from build123d import *

# Parameters (mm, degrees)
SKETCH1_R                = 49.5
BOSS_EXTRUDE1_DEPTH      = 3.18
CUT_EXTRUDE1_START       = -3.18
CUT_EXTRUDE1_DEPTH       = 3.18
CIRPATTERN1_COUNT        = 20
CUT_EXTRUDE2_DEPTH       = 70.51411196
FILLET2_R                = 1
CIRPATTERN2_COUNT        = 6
FILLET2_OF_CIRPATTERN2_R = 1
CUT_EXTRUDE3_DEPTH       = 70.51411196
SKETCH7_R                = 1
CUT_EXTRUDE4_DEPTH       = 70.51411196
CIRPATTERN3_COUNT        = 6


with BuildPart() as part:
    # Sketch1 → Boss-Extrude1 (new body)
    with BuildSketch(Plane.XY):
        with Locations(Location((0, 0, 0), (0, 0, 180))):
            Circle(SKETCH1_R)
    extrude(amount=BOSS_EXTRUDE1_DEPTH)

    # Sketch2 → Cut-Extrude1 (cut)
    with BuildSketch(Plane.XY.offset(3.18).offset(CUT_EXTRUDE1_START)):
        with BuildLine():
            ThreePointArc((-6.261015826, 49.102440681), (-3.38164679, 44.537884692), (-1.984798992, 39.324943712))
            ThreePointArc((-1.984798992, 39.324943712), (0, 39.375), (1.984798992, 39.324943712))
            ThreePointArc((1.984798992, 39.324943712), (3.38164679, 44.537884692), (6.261015826, 49.102440681))
            ThreePointArc((6.261015826, 49.102440681), (0, 49.5), (-6.261015826, 49.102440681))
        make_face()
    cut_extrude1 = extrude(amount=CUT_EXTRUDE1_DEPTH, mode=Mode.SUBTRACT)

    # CirPattern1: Cut-Extrude1 ×20 about axis
    cirpattern1_axis = Axis((0, 0, 0), (0, 0, 1))
    for i in range(1, CIRPATTERN1_COUNT):
        add(cut_extrude1.rotate(cirpattern1_axis, i * 360 / CIRPATTERN1_COUNT), mode=Mode.SUBTRACT)

    # Sketch3 → Cut-Extrude2 (cut, through all)
    with BuildSketch(Plane.XY.offset(3.18)):
        Polygon((6.06887616, 7.947876581), (29.56119168, 16.498380165), (14.619379743, 31.440192101), align=None)
    cut_extrude2 = extrude(amount=-CUT_EXTRUDE2_DEPTH, mode=Mode.SUBTRACT)

    # Fillet2
    fillet2_edges = [part.edges().sort_by_distance(p)[0] for p in [
        (29.56119168, 16.498380165, 1.59),
        (6.06887616, 7.947876581, 1.59),
        (14.619379743, 31.440192101, 1.59),
    ]]
    fillet(fillet2_edges, radius=FILLET2_R)

    # CirPattern2: Cut-Extrude2 ×6 about axis
    cirpattern2_axis = Axis((0, 0, 0), (0, 0, 1))
    for i in range(1, CIRPATTERN2_COUNT):
        add(cut_extrude2.rotate(cirpattern2_axis, i * 360 / CIRPATTERN2_COUNT), mode=Mode.SUBTRACT)

    # Fillet2 of CirPattern2
    fillet2_of_cirpattern2_edges = [part.edges().sort_by_distance(p)[0] for p in [
        (0.492579496, 33.849933043, 1.59),
        (-3.848624946, 9.229739218, 1.59),
        (-19.918315188, 28.380850296, 1.59),
        (-29.068612184, 17.351552878, 1.59),
        (-9.917501106, 1.281862636, 1.59),
        (-34.537694931, -3.059341805, 1.59),
        (-29.56119168, -16.498380165, 1.59),
        (-6.06887616, -7.947876581, 1.59),
        (-14.619379743, -31.440192101, 1.59),
        (-0.492579496, -33.849933043, 1.59),
        (3.848624946, -9.229739218, 1.59),
        (19.918315188, -28.380850296, 1.59),
        (29.068612184, -17.351552878, 1.59),
        (9.917501106, -1.281862636, 1.59),
        (34.537694931, 3.059341805, 1.59),
    ]]
    fillet(fillet2_of_cirpattern2_edges, radius=FILLET2_OF_CIRPATTERN2_R)

    # Sketch5 → Cut-Extrude3 (cut, through all)
    with BuildSketch(Plane.XY.offset(3.18)):
        with BuildLine():
            Line((-1.322875656, 1.5), (1.322875656, 1.5))
            ThreePointArc((1.322875656, 1.5), (0, -2), (-1.322875656, 1.5))
        make_face()
    extrude(amount=-CUT_EXTRUDE3_DEPTH, mode=Mode.SUBTRACT)

    # Sketch7 → Cut-Extrude4 (cut, through all)
    with BuildSketch(Plane(origin=(0, 0, 0), x_dir=(-1, 0, 0), z_dir=(0, 0, -1))):
        with Locations((-1.505042839, 10.341051496)):
            Circle(SKETCH7_R)
    cut_extrude4 = extrude(amount=-CUT_EXTRUDE4_DEPTH, mode=Mode.SUBTRACT)

    # CirPattern3: Cut-Extrude4 ×6 about axis
    cirpattern3_axis = Axis((0, 0, 0), (0, 0, 1))
    for i in range(1, CIRPATTERN3_COUNT):
        add(cut_extrude4.rotate(cirpattern3_axis, i * 360 / CIRPATTERN3_COUNT), mode=Mode.SUBTRACT)


solid = part.part
CAD build for the part. Positions are in the model's coordinates, mm. A direction names the side the tool comes from. Give positions to 0.01 mm unless a question says otherwise; leave off trailing zeros. Put each result on its own line as item: value. Start each with the question number.
(1) Probe L1, parallel to X at y = -27.5, z = 0.3; L2, parallel to Y at x = 24.5, z = 3; L3, parallel to Y at x = 21, z = 0.8. List the from-to ranges inside material, lowest first.
(2) Mould opens along X. For faces 1 (the face through (22.491, 44.095, 1.568)), 2 (the face through (-10.54, -43.48, 1.57)), 3 (the face through (-39.375, -0.028, 1.568)) say: +X half, -X half, draft (parallel to the pull), parting line (faces both ways), or undercut.
(3) Which spindle directions (+Z, -Z, +X, -X, +Y, -Y) get a long thin tool onto all of the face, cutting with end or side? Do faces 4 (the face through (-10, -1, 0)), 5 (the face through (-23.426, 37.946, 1.568)), 6 (the face through (-3.35, -44.47, 1.57)). Say none if no direction does.
(4) Flat gauge pins, fed straight in: pin 1 Ø4.5 at (x, y) = (0, 0) entering from +Z; pin 2 Ø1.5 at (y, z) = (-37, 1.5) entering from -X; pin 3 Ø0.8 at (x, z) = (-0.5, 1.5) entering from -Y. Where does each tip first touch, or does it go through?
(5) Band-saw the part on A-A, the plane z = 1.55. Give the number of separate pieces and of enclosed holes in the cut face, and give its area (3 significant figures).
Response values:
1. L1: x = -33.12 to -18.56, -13.19 to 0.63, 19.09 to 33.12
1. L2: y = -30.82 to -13.52, 1.29 to 14.66, 21.56 to 30.82
1. L3: y = -44.69 to -10.58, 0.67 to 13.38, 25.06 to 44.69
2. face 1: +X half
2. face 2: undercut
2. face 3: -X half
3. face 4: -Z, +X, -X, +Y, -Y
3. face 5: +Z, -Z
3. face 6: +Z, -Z, -Y
4. pin 1: stops at z = 3.18
4. pin 2: stops at x = -23.38
4. pin 3: stops at y = -39.37
5. separate pieces: 1
5. enclosed holes: 13
5. area: 4,800 mm2
